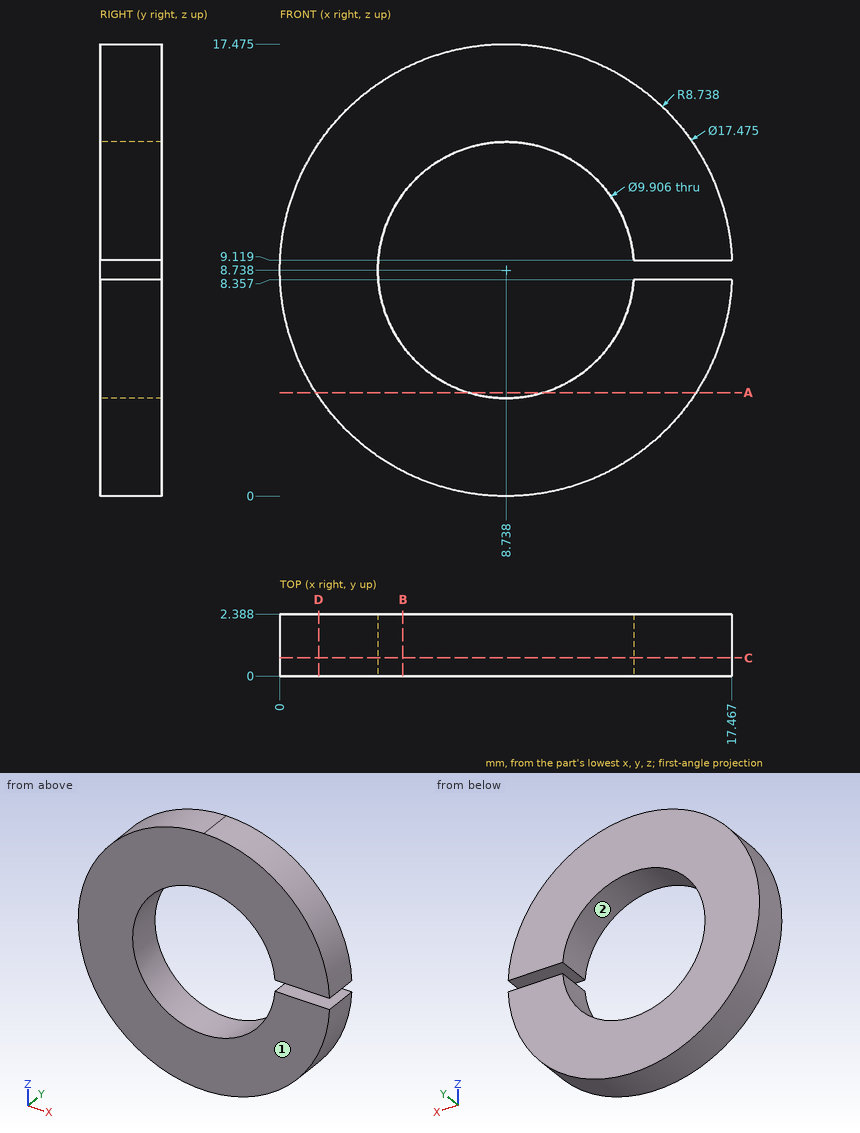
Study the drawing (mm; zero at the part's minimum x, y, z) and answer. Give positions to 0.01 mm unless a question says otherwise; leave off trailing zeros. Write each loop counter-clockwise with the first axis right and the second up, starting at its lowest first coordinate (ties: lowest second). Pieces come first, ordered by that corner, then holes. Notation, with made-up numbers: (45, 86) - (93, 86) arc R23 ccw to (93, 122) - close; hole circle Ø11 at (10.25, -36.5). An arc over 180 degrees is marked (long way). Use a Markdown table: item, result.
1. Section B-B on x = 4.75 is taken. Write down the section's boundary in (y, z) (1 decimal), plus the area to 3 significant figures.
Values follow:
| item | result |
|---|---|
| outline | (0, 1) - (2.4, 1) - (2.4, 5.8) - (0, 5.8) - close; (0, 11.7) - (2.4, 11.7) - (2.4, 16.5) - (0, 16.5) - close |
| area | 23.1 mm² |
2. Find the intervals of material crossed by probe 1 along X at (y, z) = (0.3, 7.75) (1 decimal); probe 2 along Z at (x, y) = (4.5, 1.2) (1 decimal); probe 3 along Z at (x, y) = (14, 1.85) (1 decimal), in increasing order. Write a range as from..to.
Values follow:
| item | result |
|---|---|
| probe 1 | x = 0.1..3.9, 13.6..17.4 |
| probe 2 | z = 1.1..6.2, 11.3..16.4 |
| probe 3 | z = 1.8..8.4, 9.1..15.7 |
3. Section D-D on x = 1.5 is taken. Write down the section's boundary in (y, z), plus the area to 3 significant figures.
Values follow:
| item | result |
|---|---|
| outline | (0, 3.84) - (2.39, 3.84) - (2.39, 13.63) - (0, 13.63) - close |
| area | 23.4 mm² |
4. For a pull along X with two mould halves and no side action, classify the marked faces 1 and 2 as released by +X, released by -X, zero draft, split by the parting line, or undercut.
Values follow:
| item | result |
|---|---|
| face 1 | zero draft |
| face 2 | undercut |
5. Section C-C on y = 0.7 is taken. Write down the section's boundary in (x, z) (1 decimal), plus the area to 3 significant figures.
Values follow:
| item | result |
|---|---|
| outline | (13.7, 8.4) arc R5 cw (long way) to (13.7, 9.1) - (17.5, 9.1) arc R8.7 ccw (long way) to (17.5, 8.4) - close |
| area | 160 mm² |
6. Section A-A on z = 4 is taken. Write down the section's boundary in (x, y).
Values follow:
| item | result |
|---|---|
| outline | (1.4, 0) - (7.29, 0) - (7.29, 2.39) - (1.4, 2.39) - close; (10.18, 0) - (16.08, 0) - (16.08, 2.39) - (10.18, 2.39) - close |
7. Each of these flat-tipped pins is pushed along its axis until it touches: P1, Ø5, axis at x = 7, z = 9.5, coming from the -Y side; P2, Ø0.7, axis at x = 16, y = 1, coming from the +Z side. Where does it stop, or does it pass through?
Values follow:
| item | result |
|---|---|
| P1 | passes through |
| P2 | stops at z = 14.08 |
